```python
from build123d import *

# Parameters (mm, degrees)
F1_DEPTH = 10


with BuildPart() as f1:
    # F0 (on Front) → F1 (new body)
    with BuildSketch(Plane.XZ):
        with BuildLine():
            Line((-41.2459699212, 49.2324725474), (-41.8065555243, 49.2324725474))
            ThreePointArc((-41.8065555243, 49.2324725474), (-47.0306271881, 43.9337496798), (-42.2094407409, 38.2659855689))
            Line((-42.2094407409, 38.2659855689), (-40.8129731674, 38.2698337294))
            ThreePointArc((-40.8129731674, 38.2698337294), (-37.3869527055, 40.0976581171), (-36.018184972, 43.7315311321))
            ThreePointArc((-36.018184972, 43.7315311321), (-37.5335947518, 47.5259379346), (-41.2459699212, 49.2324725474))
        make_face()
        with BuildLine():
            ThreePointArc((-41.2459699212, 49.2324725474), (-41.5262627227, 49.2396088829), (-41.8065555243, 49.2324725474))
            Line((-41.8065555243, 49.2324725474), (-41.2459699212, 49.2324725474))
        make_face()
        with BuildLine():
            Line((-40.8129731674, 38.2698337294), (-42.2094407409, 38.2659855689))
            ThreePointArc((-42.2094407409, 38.2659855689), (-41.5110845063, 38.2234742941), (-40.8129731674, 38.2698337294))
        make_face()
        with BuildLine():
            Line((19.3958776676, 49.2324725474), (-41.2459699212, 49.2324725474))
            ThreePointArc((-41.2459699212, 49.2324725474), (-37.5335947518, 47.5259379346), (-36.018184972, 43.7315311321))
            ThreePointArc((-36.018184972, 43.7315311321), (-37.3869527055, 40.0976581171), (-40.8129731674, 38.2698337294))
            Line((-40.8129731674, 38.2698337294), (20.3249844191, 38.4383078715))
            Line((20.3249844191, 38.4383078715), (20.7272791052, 38.4394164505))
            ThreePointArc((20.7272791052, 38.4394164505), (15.2765817998, 43.2456806036), (19.3958776676, 49.2324725474))
        make_face()
        with BuildLine():
            ThreePointArc((22.0284968869, 49.2324725474), (20.7121872773, 49.3930079541), (19.3958776676, 49.2324725474))
            Line((19.3958776676, 49.2324725474), (20.0357145698, 49.2324725474))
            Line((20.0357145698, 49.2324725474), (22.0284968869, 49.2324725474))
        make_face()
        with BuildLine():
            Line((20.0357145698, 49.2324725474), (19.3958776676, 49.2324725474))
            ThreePointArc((19.3958776676, 49.2324725474), (15.2765817998, 43.2456806036), (20.7272791052, 38.4394164505))
            ThreePointArc((20.7272791052, 38.4394164505), (24.5902061403, 40.0488544865), (26.1889934258, 43.9162018055))
            ThreePointArc((26.1889934258, 43.9162018055), (25.0252243831, 47.2915708983), (22.0284968869, 49.2324725474))
            Line((22.0284968869, 49.2324725474), (20.0357145698, 49.2324725474))
        make_face()
        with BuildLine():
            Line((72.3443325591, 49.2324725474), (22.0284968869, 49.2324725474))
            ThreePointArc((22.0284968869, 49.2324725474), (25.0252243831, 47.2915708983), (26.1889934258, 43.9162018055))
            ThreePointArc((26.1889934258, 43.9162018055), (24.5902061403, 40.0488544865), (20.7272791052, 38.4394164505))
            Line((20.7272791052, 38.4394164505), (69.5565042771, 38.5739721692))
            Line((69.5565042771, 38.5739721692), (69.5565042771, 44.2997200327))
            ThreePointArc((69.5565042771, 44.2997200327), (70.3016811147, 47.1327411189), (72.3443325591, 49.2324725474))
        make_face()
        with BuildLine():
            ThreePointArc((81.0534632591, 44.7649656204), (77.942418688, 49.4228865599), (72.3443325591, 49.2324725474))
            ThreePointArc((72.3443325591, 49.2324725474), (70.3016811147, 47.1327411189), (69.5565042771, 44.2997200327))
            ThreePointArc((69.5565042771, 44.2997200327), (70.993741542, 40.4937686642), (74.5879509602, 38.58783702))
            ThreePointArc((74.5879509602, 38.58783702), (78.9425359244, 39.8287087647), (81.0534632591, 43.8344744449))
            Line((81.0534632591, 43.8344744449), (81.0534632591, 44.7649656204))
        make_face()
        with BuildLine():
            Line((69.5565042771, 44.2997200327), (69.5565042771, 38.5739721692))
            Line((69.5565042771, 38.5739721692), (74.5879509602, 38.58783702))
            ThreePointArc((74.5879509602, 38.58783702), (70.993741542, 40.4937686642), (69.5565042771, 44.2997200327))
        make_face()
        with BuildLine():
            Line((74.5879509602, 38.58783702), (69.5565042771, 38.5739721692))
            Line((69.5565042771, 38.5739721692), (69.5565042771, -41.8843869054))
            Line((69.5565042771, -41.8843869054), (77.41492293, -41.8627319403))
            ThreePointArc((77.41492293, -41.8627319403), (77.8187709933, -41.8492012292), (78.2226874942, -41.8605060327))
            ThreePointArc((78.2226874942, -41.8605060327), (79.6851867949, -42.1143399773), (81.0534632591, -42.689801004))
            Line((81.0534632591, -42.689801004), (81.0534632591, 43.8344744449))
            ThreePointArc((81.0534632591, 43.8344744449), (78.9425359244, 39.8287087647), (74.5879509602, 38.58783702))
        make_face()
        with BuildLine():
            ThreePointArc((81.0722902774, 44.2997200327), (81.0675815975, 44.5325332161), (81.0534632591, 44.7649656204))
            Line((81.0534632591, 44.7649656204), (81.0534632591, 43.8344744449))
            ThreePointArc((81.0534632591, 43.8344744449), (81.0675815975, 44.0669068492), (81.0722902774, 44.2997200327))
        make_face()
        with BuildLine():
            Line((77.41492293, -41.8627319403), (69.5565042771, -41.8843869054))
            Line((69.5565042771, -41.8843869054), (25.4644663722, -42.005888646))
            ThreePointArc((25.4644663722, -42.005888646), (27.4470484848, -44.5675644173), (28.1525257136, -47.7290698293))
            ThreePointArc((28.1525257136, -47.7290698293), (26.1341587579, -52.8227999815), (21.1746559331, -55.1515815863))
            Line((21.1746559331, -55.1515815863), (77.680068251, -54.9958730667))
            ThreePointArc((77.680068251, -54.9958730667), (71.2639429971, -48.556161307), (77.41492293, -41.8627319403))
        make_face()
        with BuildLine():
            Line((78.2226874942, -41.8605060327), (77.41492293, -41.8627319403))
            ThreePointArc((77.41492293, -41.8627319403), (71.2639429971, -48.556161307), (77.680068251, -54.9958730667))
            Line((77.680068251, -54.9958730667), (78.0299260429, -54.9949089849))
            ThreePointArc((78.0299260429, -54.9949089849), (82.5533635979, -53.0034225515), (84.4111709763, -48.4234599673))
            ThreePointArc((84.4111709763, -48.4234599673), (83.5099767883, -45.1012225352), (81.0534632591, -42.689801004))
            ThreePointArc((81.0534632591, -42.689801004), (79.6851867949, -42.1143399773), (78.2226874942, -41.8605060327))
        make_face()
        with BuildLine():
            ThreePointArc((28.1525257136, -47.7290698293), (27.4470484848, -44.5675644173), (25.4644663722, -42.005888646))
            ThreePointArc((25.4644663722, -42.005888646), (23.4623029685, -40.8181243584), (21.1910051796, -40.3075867475))
            Line((21.1910051796, -40.3075867475), (20.3734561107, -40.3002775684))
            ThreePointArc((20.3734561107, -40.3002775684), (13.2791728637, -47.7368050161), (20.3889108114, -55.1585582849))
            Line((20.3889108114, -55.1585582849), (21.1746559331, -55.1515815863))
            ThreePointArc((21.1746559331, -55.1515815863), (26.1341587579, -52.8227999815), (28.1525257136, -47.7290698293))
        make_face()
        with BuildLine():
            Line((78.0299260429, -54.9949089849), (77.680068251, -54.9958730667))
            ThreePointArc((77.680068251, -54.9958730667), (77.8550035612, -54.9977187055), (78.0299260429, -54.9949089849))
        make_face()
        with BuildLine():
            Line((20.3734561107, -40.3002775684), (21.1910051796, -40.3075867475))
            ThreePointArc((21.1910051796, -40.3075867475), (20.7823311667, -40.2926885818), (20.3734561107, -40.3002775684))
        make_face()
        with BuildLine():
            ThreePointArc((20.3889108114, -55.1585582849), (20.7818755833, -55.1654551359), (21.1746559331, -55.1515815863))
            Line((21.1746559331, -55.1515815863), (20.3889108114, -55.1585582849))
        make_face()
        with BuildLine():
            ThreePointArc((20.3889108114, -55.1585582849), (13.2791728637, -47.7368050161), (20.3734561107, -40.3002775684))
            Line((20.3734561107, -40.3002775684), (-41.3835467647, -39.7481480292))
            ThreePointArc((-41.3835467647, -39.7481480292), (-35.8317624102, -42.1354889714), (-33.5440649914, -47.7290698293))
            ThreePointArc((-33.5440649914, -47.7290698293), (-34.1207054737, -50.7078619424), (-35.7673129619, -53.2562733061))
            ThreePointArc((-35.7673129619, -53.2562733061), (-38.2588759048, -55.0119033441), (-41.226844648, -55.7056498884))
            Line((-41.226844648, -55.7056498884), (20.3889108114, -55.1585582849))
        make_face()
        with BuildLine():
            Line((-41.5262627227, -39.7468720979), (-41.3835467647, -39.7481480292))
            ThreePointArc((-41.3835467647, -39.7481480292), (-41.454901892, -39.7471910871), (-41.5262627227, -39.7468720979))
        make_face()
        with BuildLine():
            ThreePointArc((-33.5440649914, -47.7290698293), (-35.8317624102, -42.1354889714), (-41.3835467647, -39.7481480292))
            Line((-41.3835467647, -39.7481480292), (-41.5262627227, -39.7468720979))
            ThreePointArc((-41.5262627227, -39.7468720979), (-49.5080707965, -47.6501997041), (-41.6839952729, -55.7097089682))
            Line((-41.6839952729, -55.7097089682), (-35.7673129619, -53.2562733061))
            ThreePointArc((-35.7673129619, -53.2562733061), (-34.1207054737, -50.7078619424), (-33.5440649914, -47.7290698293))
        make_face()
        with BuildLine():
            Line((-41.6839952729, -55.7097089682), (-41.226844648, -55.7056498884))
            ThreePointArc((-41.226844648, -55.7056498884), (-38.2588759048, -55.0119033441), (-35.7673129619, -53.2562733061))
            Line((-35.7673129619, -53.2562733061), (-41.6839952729, -55.7097089682))
        make_face()
        with BuildLine():
            ThreePointArc((-41.6839952729, -55.7097089682), (-41.4553908947, -55.7109529283), (-41.226844648, -55.7056498884))
            Line((-41.226844648, -55.7056498884), (-41.6839952729, -55.7097089682))
        make_face()
    extrude(amount=F1_DEPTH)


solid = f1.part
```
Source: CAD feature listing. Evaluate the final solid. Frame: model axes, mm. A direction names the side the tool comes from. Give positions to 0.01 mm unless a question says otherwise; leave off trailing zeros. Loops run counter-clockwise (first coordinate to the right, second up) from the corner with the lowest first, then second, coordinate; pieces in that order, holes last. Notation, with made-up numbers: (-16.5, 25) -> (27.5, 25) arc R29 ccw to (27.5, 53) -> close; hole circle Ø6 at (72.25, 43.25). An arc over 180 degrees is marked (long way). Put each result on its own line as item: value. Start each with the question number.
1) Cut plane A-A (x = 62.5). Return loops of the section in (y, z).
2) Reachability of faces 5 (the face through (-11, -5, 49.232)), 6 (the face through (22, 0, -42)) from +Z, -Z, +X, -X, +Y, -Y: full face, straight path, thin tool, end or side. Return the list, or none.
3) Draft query along X for faces 1 (the face through (22, -10, -42)), 2 (the face through (48, -5, 49.232)), 3 (the face through (81.053, -5, 0)), 4 (the face through (20.731, -4.93, 49.393)). Return one class per face: released by +X, released by -X, zero draft, split by the parting line, or undercut.
4) Material intervals for probe 1 along Z at (x, y) = (-40, -7.75); probe 2 along Z at (x, y) = (27, -2.5); probe 3 along X at (y, z) = (-9.25, -37), sorted ascending.
5) Cut plane C-C (x = 48.5). Return loops of the section in (y, z).
6) Cut plane D-D (z = 40). Return loops of the section in (x, y).
7) Contact query for flat-ended pins moving along their axis: P1, Ø6, axis at x = 55.5, y = -2.5, coming from the -Z side; P2, Ø5, axis at y = -7, z = -4, coming from the +X side; P3, Ø5, axis at x = 41, y = -2.5, coming from the +Z side; P4, Ø12, axis at x = 65.5, z = -42, coming from the +Y side. Output: stop coordinate, or through.
8) Cut plane B-B (y = -3.75). Return loops of the section in (x, z).
Results are:
1. outline: (-10, -55.04) -> (0, -55.04) -> (0, -41.9) -> (-10, -41.9) -> close; (-10, 38.55) -> (0, 38.55) -> (0, 49.23) -> (-10, 49.23) -> close
2. face 5: +Z, -X, +Y, -Y
2. face 6: +Z, -Z, +X, -X, +Y
3. face 1: zero draft
3. face 2: undercut
3. face 3: released by +X
3. face 4: undercut
4. probe 1: z = -55.69 to -39.76, 38.27 to 49.23
4. probe 2: z = -55.14 to -42, 38.46 to 49.23
4. probe 3: x = 69.56 to 81.05
5. outline: (-10, -55.08) -> (0, -55.08) -> (0, -41.94) -> (-10, -41.94) -> close; (-10, 38.52) -> (0, 38.52) -> (0, 49.23) -> (-10, 49.23) -> close
6. outline: (-45.58, -10) -> (81.05, -10) -> (81.05, 0) -> (-45.58, 0) -> close
7. P1: stops at z = -55.07
7. P2: stops at x = 81.05
7. P3: stops at z = 49.23
7. P4: stops at y = 0
8. outline: (-41.38, -39.75) arc R7.98 ccw (long way) to (-41.23, -55.71) -> (20.39, -55.16) arc R7.44 ccw to (21.17, -55.15) -> (77.68, -55) arc R6.57 ccw to (81.05, -42.69) -> (81.05, 43.83) arc R5.76 ccw to (72.34, 49.23) -> (22.03, 49.23) arc R5.48 ccw to (19.4, 49.23) -> (-41.25, 49.23) arc R5.51 ccw (long way) to (-40.81, 38.27) -> (69.56, 38.57) -> (69.56, -41.88) -> (25.46, -42.01) arc R7.44 ccw to (20.37, -40.3) -> close; hole (77.41, -41.86) -> (78.22, -41.86) arc R6.57 ccw to start
